from build123d import *

# Parameters (mm, degrees)
SKETCH1_R               = 84.1375
SKETCH1_R_2             = 77.0255
EXTRUDE1_DEPTH          = 25.4
CHAMFER1_SIZE           = 7.62
CHAMFER1_SIZE2          = 5.847031648
CUT_EXTRUDE1_DEPTH      = 122.669214728
CUT_EXTRUDE2_DEPTH      = 122.669214887
CUT_EXTRUDE2_DEPTH_BACK = 122.669214887


with BuildPart() as part:
    # Sketch1 → Extrude1 (new, symmetric)
    with BuildSketch(Plane.XY):
        Circle(SKETCH1_R)
        Circle(SKETCH1_R_2, mode=Mode.SUBTRACT)
    extrude(amount=EXTRUDE1_DEPTH, both=True)

    # Chamfer1
    chamfer1_edges = [part.edges().sort_by_distance(p)[0] for p in [
        (-84.1375, 0, 25.4),
    ]]
    chamfer1_side = [part.faces().sort_by_distance(p)[0] for p in [
        (-84.1375, 0, 0),
    ]]
    chamfer(chamfer1_edges, length=CHAMFER1_SIZE, length2=CHAMFER1_SIZE2, reference=chamfer1_side[0])

    # Sketch2 → Cut-Extrude1 (cut, through all)
    with BuildSketch(Plane(origin=(0, 0, 0), x_dir=(0, 0, -1), z_dir=(1, 0, 0))):
        with BuildLine():
            Line((25.4, 84.1375), (25.4, -84.1375))
            ThreePointArc((25.4, -84.1375), (9.353148868, 0), (25.4, 84.1375))
        make_face()
    extrude(amount=-CUT_EXTRUDE1_DEPTH, mode=Mode.SUBTRACT)

    # Sketch2<2> → Cut-Extrude2 (cut, two sides: drawn at the far end of the back side and taken through both)
    with BuildSketch(Plane(origin=(0, 0, 0), x_dir=(0, 0, -1), z_dir=(1, 0, 0)).offset(-CUT_EXTRUDE2_DEPTH_BACK)):
        with BuildLine():
            Line((25.4, 84.1375), (25.4, -84.1375))
            ThreePointArc((25.4, -84.1375), (9.353148868, 0), (25.4, 84.1375))
        make_face()
    extrude(amount=CUT_EXTRUDE2_DEPTH + CUT_EXTRUDE2_DEPTH_BACK, mode=Mode.SUBTRACT)


solid = part.part
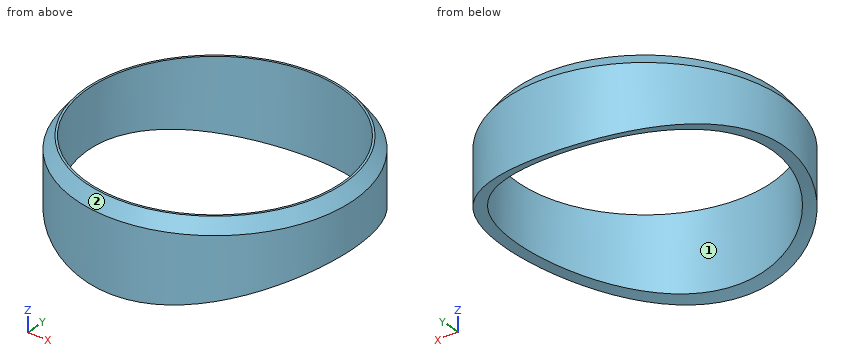
Verification items for the finished model (mm, model axes). Face numbers are marked on the shaded views. Coordinates: 2 decimals unless noted, no trailing zeros. Loops run counter-clockwise (first coordinate to the right, second up) from the corner with the lowest first, then second, coordinate; pieces in that order, holes last. Notation, with made-up numbers: (88.5, 55) -> (141.5, 55) arc R21 ccw to (141.5, 67) -> close; hole circle Ø1 at (72.5, 48). An arc over 180 degrees is marked (long way). Answer as CSV lines item,"result".
1) Release check for a two-part mould opening along X. For the marked faces 1 and 2 record: +X half, -X half, draft (parallel to the pull), parting line (faces both ways), or undercut.
Found:
face 1,"undercut"
face 2,"parting line"
2) Depth check by flat-ended pin: pin 1 (5 mm diameter, centred on x = 8.5, z = -15.5, fed in from +Y); pin 2 (8 mm diameter, centred on x = 34.5, z = -15.5, fed in from +Y); pin 3 (1 mm diameter, centred on x = 46, z = -14.5, fed in from +Y). Enter the tip coordinate at first touch or a pass-through.
Found:
pin 1,"stops at y = 83.92"
pin 2,"stops at y = 78.41"
pin 3,"stops at y = 70.77"
3) Cross-section at B-B, the plane x = 0. Record the cut outline in (y, z).
Found:
outline,"(-84.14, -25.4) arc R228.6 cw to (-77.03, -22.72) -> (-77.03, 25.4) -> (-78.29, 25.4) -> (-84.14, 17.78) -> close; (77.03, -22.72) arc R228.6 cw to (84.14, -25.4) -> (84.14, 17.78) -> (78.29, 25.4) -> (77.03, 25.4) -> close"
4) Cross-section at D-D, the plane z = 12. Record the cut outline in (x, y) (1 decimal).
Found:
outline,"circle Ø168.3 at (0, 0); hole circle Ø154.1 at (0, 0)"
5) Cross-section at C-C, the plane z = -18. Record the cut outline in (x, y) (1 decimal).
Found:
outline,"(-56.6, -62.3) arc R84.1 ccw to (56.6, -62.3) -> (45.3, -62.3) arc R77 cw to (-45.3, -62.3) -> close; (-56.6, 62.3) -> (-45.3, 62.3) arc R77 cw to (45.3, 62.3) -> (56.6, 62.3) arc R84.1 ccw to start"
6) Cross-section at A-A, the plane y = 0. Record the cut outline in (x, z), then the cut area to 3 significant figures.
Found:
outline,"(-84.14, -9.35) -> (-77.03, -9.35) -> (-77.03, 25.4) -> (-78.29, 25.4) -> (-84.14, 17.78) -> close; (77.03, -9.35) -> (84.14, -9.35) -> (84.14, 17.78) -> (78.29, 25.4) -> (77.03, 25.4) -> close"
area,"450 mm2"
7) Thickness scan on L1, parallel to X at y = 0, z = 2; L2, parallel to Y at x = -36, z = 9.5. Record the ranges inside material, lowest first. Write a range as from..to.
Found:
L1,"x = -84.14..-77.03, 77.03..84.14"
L2,"y = -76.05..-68.09, 68.09..76.05"
